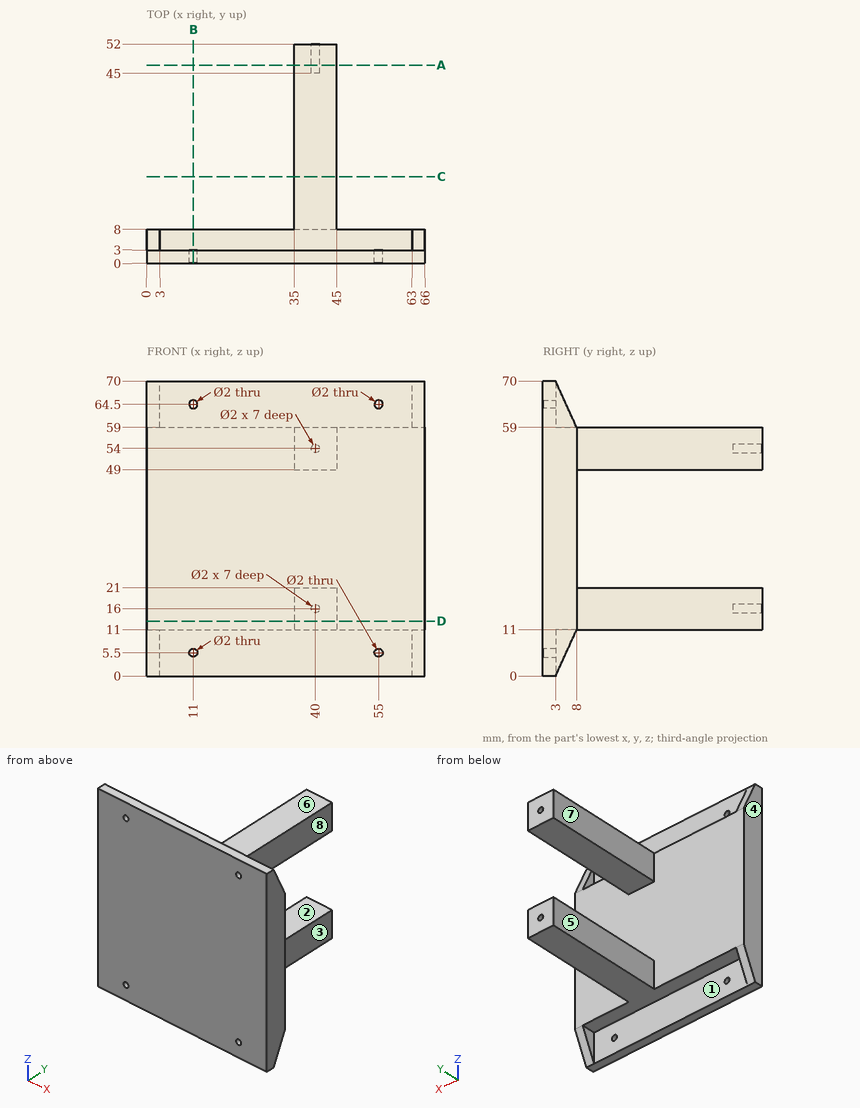
Drawing for the job (mm, zero at the part's lowest x, y, z). A direction names the side the tool comes from. Round coordinates to 2 decimals unless told otherwise and drop trailing zeros. Order: outer loops, then holes, each group sorted by start corner. A loop starts at its lowest first (then second) coordinate and runs counter-clockwise, first axis right, second up. Notation, with made-up numbers: (46.5, 3) -> (83.5, 3) arc R23 cw to (83.5, 13) -> close; hole circle Ø10 at (50, 34). An arc over 180 degrees is marked (long way). Write item = value, one per line. Start each with the question number.
(1) Pull direction X, two halves, no side cores. Call the marked faces 6, 7 and 8: released by +X, released by -X, zero draft, split by the parting line, or undercut.
(2) Pin check, flat tips, straight feed: P1, Ø4, axis at x = 41.5, y = 19.5, coming from the +Z side; P2, Ø3, axis at x = 40, z = 16, coming from the -Y side; P3, Ø0.6, axis at x = 40, z = 54.5, coming from the +Y side; P4, Ø24.5, axis at x = 29.5, y = 36, coming from the -Z side. Stop position of each tip, or through.
(3) Which spindle directions (+Z, -Z, +X, -X, +Y, -Y) get a long thin tool onto all of the face, cutting with end or side? Do the marked faces 1, 2, 3, 4 and 5. Say none if no direction does.
(4) Probe line 1 (X direction, y = 0.7, z = 64.5); line 2 (Z direction, x = 37, y = 43.5); line 3 (Y direction, x = 21.5, z = 53). List the from-to ranges inside material, lowest first. Write a range as [from, to].
(5) Cut at C-C, the plane y = 20.5. List the corners of the cut face in (x, z).
(6) Cut at B-B, the plane x = 11. List the corners of the cut face in (y, z).
(7) Cut at D-D, the plane z = 13. List the corners of the cut face in (x, y).
(8) Cut at A-A, the plane y = 47. List the corners of the cut face in (x, z).
Model answer:
q1.face_6 = undercut
q1.face_7 = released by -X
q1.face_8 = released by +X
q2.P1 = 59
q2.P2 = 0
q2.P3 = 45
q2.P4 = 11
q3.face_1 = -Z, +Y
q3.face_2 = +X, -X, +Y
q3.face_3 = +Z, -Z, +X, +Y
q3.face_4 = +Z, -Z, -X, +Y, -Y
q3.face_5 = +Z, -Z, -X, +Y
q4.line_1 = [0, 10], [12, 54], [56, 66]
q4.line_2 = [11, 21], [49, 59]
q4.line_3 = [0, 8]
q5.outline = (35, 11) -> (45, 11) -> (45, 21) -> (35, 21) -> close; (35, 49) -> (45, 49) -> (45, 59) -> (35, 59) -> close
q6.outline = (0, 0) -> (3, 0) -> (3, 4.5) -> (0, 4.5) -> close; (0, 6.5) -> (3, 6.5) -> (3, 11) -> (8, 11) -> (8, 59) -> (3, 59) -> (3, 63.5) -> (0, 63.5) -> close; (0, 65.5) -> (3, 65.5) -> (3, 70) -> (0, 70) -> close
q7.outline = (0, 0) -> (66, 0) -> (66, 8) -> (45, 8) -> (45, 52) -> (35, 52) -> (35, 8) -> (0, 8) -> close
q8.outline = (35, 11) -> (45, 11) -> (45, 21) -> (35, 21) -> close; (35, 49) -> (45, 49) -> (45, 59) -> (35, 59) -> close; hole circle Ø2 at (40, 16); hole circle Ø2 at (40, 54)
